```python
from build123d import *

# Parameters (mm, degrees)
SKETCH1_R           = 1.5875
SKETCH1_R_2         = 1.1303
BOSS_EXTRUDE1_DEPTH = 7.14375
SKETCH2_R           = 1.5875
CUT_EXTRUDE1_DEPTH  = 0.79375


with BuildPart() as part:
    # Sketch1 → Boss-Extrude1 (new body)
    with BuildSketch(Plane.XY):
        Polygon((6.35, 1.5875), (9.525, 1.5875), (9.525, 4.224628752), (9.525, 10.562648806), (7.319307862, 9.683908365), (-11.458663934, 2.097115291), (-11.458663934, -3.175), (9.525, -3.175), (9.525, -1.5875), (6.35, -1.5875), align=None)
        Circle(SKETCH1_R, mode=Mode.SUBTRACT)
        with Locations((-8.918663934, -0.301005903)):
            Circle(SKETCH1_R_2, mode=Mode.SUBTRACT)
        with Locations((5.588425528, 5.5602387)):
            Circle(SKETCH1_R_2, mode=Mode.SUBTRACT)
    extrude(amount=BOSS_EXTRUDE1_DEPTH)

    # Sketch2 → Cut-Extrude1 (cut)
    with BuildSketch(Plane.XY):
        with BuildLine():
            Line((9.525, 1.5875), (6.148361062, 1.5875))
            ThreePointArc((6.148361062, 1.5875), (5.169946467, 3.687025023), (3.503620258, 5.29595554))
            Line((3.503620258, 5.29595554), (2.515012001, 7.742846841))
            Line((2.515012001, 7.742846841), (-8.224002276, 3.404003433))
            Line((-8.224002276, 3.404003433), (-5.565912349, -3.175))
            Line((-5.565912349, -3.175), (9.525, -3.175))
            Line((9.525, -3.175), (9.525, 1.5875))
        make_face()
        Circle(SKETCH2_R, mode=Mode.SUBTRACT)
    extrude(amount=CUT_EXTRUDE1_DEPTH, mode=Mode.SUBTRACT)


solid = part.part
```
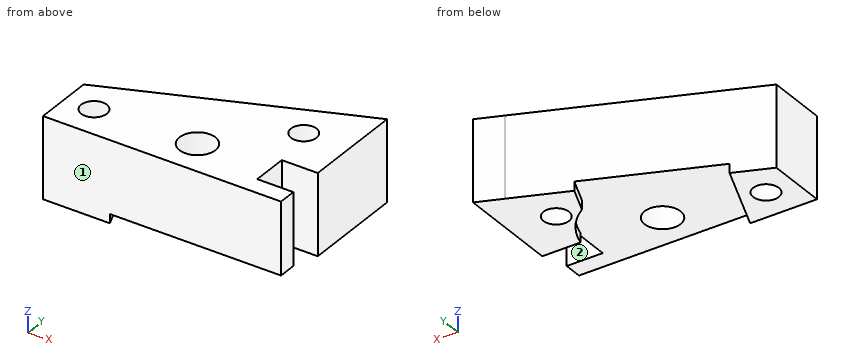
For this review, take the finished solid that the model builds, in its own axes (mm). Face numbers are marked on the shaded views. A direction names the side the tool comes from. Coordinates: 2 decimals unless noted, no trailing zeros. Loops run counter-clockwise (first coordinate to the right, second up) from the corner with the lowest first, then second, coordinate; pieces in that order, holes last. Notation, with made-up numbers: (53, -11.5) -> (92, -11.5) arc R31 cw to (92, 21.5) -> close; hole circle Ø4 at (43, 60). An arc over 180 degrees is marked (long way). Return JSON: item names as keys, results as strings. Group by question number.
(1) Consider section A-A, the plane x = 0.5. Give the boundary of the cut face in (y, z) (3 decimals).
(2) Tool access review of the marked faces 1 and 2: name each direction out of +Z, -Z, +X, -X, +Y, -Y from which nothing blocks a thin tool from reaching the whole face with its end or side.
(3) Consider section C-C, the plane z = 2.5. Count the separate pieces of the cut face and the enclosed holes in it, plus the area to 3 significant figures.
(4) Consider section B-B, the plane y = 0. Give the boundary of the cut face in (x, z), plus the area to 3 significant figures.
(5) To check wall thickness, follow L1, parallel to Y at x = 6.5, z = 1.25 (1 decimal); L2, parallel to Y at x = 7.75, z = 1.5 (1 decimal); L3, parallel to Y at x = 6, z = 3.75 (3 decimals). State the ranges of each line that lie inside material, in increasing order.
(6) Consider section D-D, the plane y = 2.75. Give the boundary of the cut face in (x, z) (3 decimals), plus the area to 3 significant figures.
(7) For pin 1 Ø1.8 at (x, y) = (5.59, 5.56) entering from +Z; pin 2 Ø3 at (x, y) = (-5, 3) entering from -Z; pin 3 Ø4 at (y, z) = (6.5, 3.5) entering from -X; pin 4 Ø4 at (y, z) = (8, 3.5) entering from -X, all flat-tipped, find the tip position at first contact; note any pin that passes through.
Results below:
{
 "1": {"outline": "(-3.175, 0.794) -> (-1.507, 0.794) -> (-1.507, 7.144) -> (-3.175, 7.144) -> close; (1.507, 0.794) -> (6.929, 0.794) -> (6.929, 7.144) -> (1.507, 7.144) -> close"},
 "2": {"face 1": "+Z, -Z, +X, -X, -Y", "face 2": "+Z, -Z, +X"},
 "3": {"separate pieces": "1", "enclosed holes": "3", "area": "174 mm2"},
 "4": {"outline": "(-11.46, 0) -> (-10.01, 0) -> (-10.01, 7.14) -> (-11.46, 7.14) -> close; (-7.83, 0) -> (-6.85, 0) -> (-6.85, 0.79) -> (-1.59, 0.79) -> (-1.59, 7.14) -> (-7.83, 7.14) -> close; (1.59, 0.79) -> (6.35, 0.79) -> (6.35, 7.14) -> (1.59, 7.14) -> close", "area": "81.0 mm2"},
 "5": {"L1": "y = -3.2 to -1.6, 1.6 to 4.9, 6.2 to 9.4", "L2": "y = -3.2 to -1.6, 1.6 to 9.9", "L3": "y = -3.175 to 4.508, 6.613 to 9.151"},
 "6": {"outline": "(-9.843, 0) -> (-7.96, 0) -> (-7.96, 0.794) -> (5.724, 0.794) -> (5.724, 0) -> (9.525, 0) -> (9.525, 7.144) -> (-9.843, 7.144) -> close", "area": "127 mm2"},
 "7": {"pin 1": "passes through", "pin 2": "stops at z = 0.79", "pin 3": "stops at x = -5.51", "pin 4": "stops at x = -1.8"}
}
